from build123d import *

# Parameters (mm, degrees)
F0_R     = 126.1012102306
F1_DEPTH = 106.68
F2_D     = 203.2
F3_DEPTH = 150.368


with BuildPart() as f1:
    # F0 (on Top) → F1 (new body)
    with BuildSketch(Plane.XY):
        Circle(F0_R)
    extrude(amount=F1_DEPTH)

    # F2 (through all)
    with Locations(Plane(origin=(0, 0, 0), x_dir=(1, 0, 0), z_dir=(0, 0, -1))):
        with Locations((0, 0)):
            Hole(F2_D / 2)

    # F3 (add): a face of the model
    f3_faces = [f1.faces().sort_by_distance(p)[0] for p in [
        (-122.5345293958, 0, 106.68),
    ]]
    extrude(f3_faces, amount=F3_DEPTH)


solid = f1.part
Model file for the job. Use its own axes, mm. Give positions to 0.01 mm unless a question says otherwise; leave off trailing zeros. Order: outer loops, then holes, each group sorted by start corner. A loop starts at its lowest first (then second) coordinate and runs counter-clockwise, first axis right, second up. Notation, with made-up numbers: (7.5, 61.5) - (28.5, 61.5) arc R14 ccw to (28.5, 82.5) - close; hole circle Ø1 at (-7.75, 47.25). An arc over 180 degrees is marked (long way). Return JSON: item names as keys, results as strings.
1) Cut at A-A, the plane y = 0. Give the cut face in (x, z), plus the area to 3 significant figures.
Geometry says:
{"outline": "(-126.1, 0) - (-101.6, 0) - (-101.6, 257.05) - (-126.1, 257.05) - close; (101.6, 0) - (126.1, 0) - (126.1, 257.05) - (101.6, 257.05) - close", "area": "12,600 mm²"}
2) Probe line 1 (Y direction, x = 0, z = 23.5); line 2 (Y direction, x = -24, z = 163); line 3 (X direction, y = 69, z = 94). List the from-to ranges inside material, lowest first. Write a range as from..to.
Geometry says:
{"line 1": "-126.1..-101.6, 101.6..126.1", "line 2": "-123.8..-98.72, 98.72..123.8", "line 3": "-105.55..-74.58, 74.58..105.55"}
3) Cut at C-C, the plane z = 57. Give the cut face in (x, y).
Geometry says:
{"outline": "circle Ø252.2 at (0, 0); hole circle Ø203.2 at (0, 0)"}
4) Cut at D-D, the plane y = 109. Give the cut face in (x, z).
Geometry says:
{"outline": "(-63.41, 0) - (63.41, 0) - (63.41, 257.05) - (-63.41, 257.05) - close"}
5) Flat gauge pins, fed straight in: P1, Ø3, axis at x = -52, z = 225, coming from the -Y side; P2, Ø10, axis at x = 39, z = 229, coming from the +Y side; P3, Ø8, axis at y = 100.5, z = 141, coming from the -X side. Where does each tip first touch, or does it go through?
Geometry says:
{"P1": "y = -115.55", "P2": "y = 121.43", "P3": "x = -81.17"}
